Verification items for the finished model (mm, model axes). A direction names the side the tool comes from. Coordinates: 2 decimals unless noted, no trailing zeros. Order: outer loops, then holes, each group sorted by start corner. A loop starts at its lowest first (then second) coordinate and runs counter-clockwise, first axis right, second up. Notation, with made-up numbers: M -36.5,42 L -5.5,42 A27 cw -5.5,61 Z; hole C 21,-33.5 d1. An arc over 180 degrees is marked long. Use one line per item in the form item = value. Start each with the question number.
Autodesk Inventor part; units mm, degrees
ref_plane "YZ Plane" through (0, 0, 0) normal (1, 0, 0) x (0, 1, 0)
ref_plane "XZ Plane" through (0, 0, 0) normal (0, 1, 0) x (-1, 0, 0)
ref_plane "XY Plane" through (0, 0, 0) normal (0, 0, 1) x (1, 0, 0)
sketch "Sketch1" plane through (0, 0, 0) normal (0, 0, 1) x (1, 0, 0)
  line L0 (0, 0) -> (25.4, 0)
  line L1 (25.4, 0) -> (25.4, 101.6)
  line L2 (25.4, 101.6) -> (0, 101.6)
  line L3 (0, 101.6) -> (0, 0)
  arc A0 (25.4, 76.2) -> (25.4, 101.6) centre (25.4, 88.9) ccw
  dimension "d0" = 101.6
  dimension "d1" = 25.4
  dimension "d2" = 25.4
extrude "Extrusion1" add sketch "Sketch1" along normal blind 3.175
sketch "Sketch4" plane through (0, 0, 3.175) normal (0, 0, 1) x (1, 0, 0)
  line L0 (25.4, 0) -> (25.4, 76.2)
  arc A0 (25.4, 76.2) -> (25.4, 101.6) centre (25.4, 88.9) ccw
  point P0 (0, 0)
hole "Hole2" at (25.4, 88.9, 3.175) direction (0, 0, -1) diameter 6.7564 end through all
fillet "Fillet1" radius 9.525 1 edges at (0, 101.6, 1.5875)
sketch "Sketch6" plane through (0, 0, 0) normal (0, 0, -1) x (-1, 0, 0)
  line L0 (-9.525, 101.6) -> (-25.4, 101.6)
  line L1 (0, 92.075) -> (0, 0)
  point P0 (-12.7, 50.8)
  dimension "d52" = 50.8
  dimension "d63" = 12.7
hole "Hole3" at (12.7, 50.8, 0) direction (0, 0, 1) diameter 4.8514 end through all countersink diameter 9.525 countersink angle 82
pattern_linear "Rectangular Pattern1" count 4 spacing 12.7 along (0, -1, 0) of "Hole3"
equation "\"d2\" = d1"
properties part number "CLB_027_LifterBracketLeft" material "Aluminum 6061"
1. Tool access check on faces 1 (the conical face through (14.438, 36.204, 2.52)), 2 (the flat face through (25.4, 38, 2)). Record the directions out of +Z, -Z, +X, -X, +Y, -Y that give a thin tool (end or side, any length) a straight path to the whole face; none if there is none.
2. Material ranges on line 1 along Y through (x, z) = (12.7, 3.05); line 2 along X through (y, z) = (88.9, 1.15); line 3 along X through (y, z) = (50.8, 3), recorded low to high.
3. Cross-section at C-C on z = 1.9. Enter the section's corners in (x, y) (3 decimals), and give its area (3 significant figures).
4. Cross-section at B-B on y = 88.9. Enter the section's corners in (x, z) (3 decimals), and give its area (3 significant figures).
5. Release check for a two-part mould opening along X. For faces 3 (the cylindrical face through (13.63, 14.94, 2.93)), 4 (the flat face through (15, 63, 0)), 5 (the cylindrical face through (38.097, 89.179, 1.565)) record: pulls with the +X half, pulls with the -X half, needs draft (parallel to the pull), parting line crosses it, or undercut.
6. Cross-section at A-A on x = 12.7. Enter the section's corners in (y, z) (1 decimal).
7. Depth check by flat-ended pin: P1, Ø5.5, axis at x = 12.7, y = 25.4, coming from the -Z side; P2, Ø4, axis at x = 12.7, y = 38.1, coming from the -Z side; P3, Ø1, axis at y = 78, z = 0.5, coming from the +X side; P4, Ø1, axis at x = 26.5, z = 1, coming from the +Y side. Enter the tip coordinate at first touch or a pass-through.
8. Cross-section at D-D on y = 12.7. Enter the section's corners in (x, z) (1 decimal).
Final values:
q1.face_1 = -Z
q1.face_2 = +Z, -Z, +X, -Y
q2.line_1 = 0 to 10.27, 15.13 to 22.97, 27.83 to 35.67, 40.53 to 48.37, 53.23 to 101.6
q2.line_2 = 0 to 22.02, 28.78 to 38.1
q2.line_3 = 0 to 10.27, 15.13 to 25.4
q3.outline = M 0,0 L 25.4,0 L 25.4,76.2 A12.7 ccw 25.4,101.6 L 9.525,101.6 A9.525 ccw 0,92.075 Z; hole C 12.7,12.7 d6.222; hole C 12.7,25.4 d6.222; hole C 12.7,38.1 d6.222; hole C 12.7,50.8 d6.222; hole C 25.4,88.9 d6.756
q3.area = 2,660 mm2
q4.outline = M 0,0 L 22.022,0 L 22.022,3.175 L 0,3.175 Z; M 28.778,0 L 38.1,0 L 38.1,3.175 L 28.778,3.175 Z
q4.area = 99.5 mm2
q5.face_3 = undercut
q5.face_4 = needs draft
q5.face_5 = pulls with the +X half
q6.outline = M 0,0 L 7.9,0 L 10.3,2.7 L 10.3,3.2 L 0,3.2 Z; M 15.1,2.7 L 17.5,0 L 20.6,0 L 23,2.7 L 23,3.2 L 15.1,3.2 Z; M 27.8,2.7 L 30.2,0 L 33.3,0 L 35.7,2.7 L 35.7,3.2 L 27.8,3.2 Z; M 40.5,2.7 L 42.9,0 L 46,0 L 48.4,2.7 L 48.4,3.2 L 40.5,3.2 Z; M 53.2,2.7 L 55.6,0 L 101.6,0 L 101.6,3.2 L 53.2,3.2 Z
q7.P1 = 2.32
q7.P2 = through
q7.P3 = 32.69
q7.P4 = 101.59
q8.outline = M 0,0 L 7.9,0 L 10.3,2.7 L 10.3,3.2 L 0,3.2 Z; M 15.1,2.7 L 17.5,0 L 25.4,0 L 25.4,3.2 L 15.1,3.2 Z
